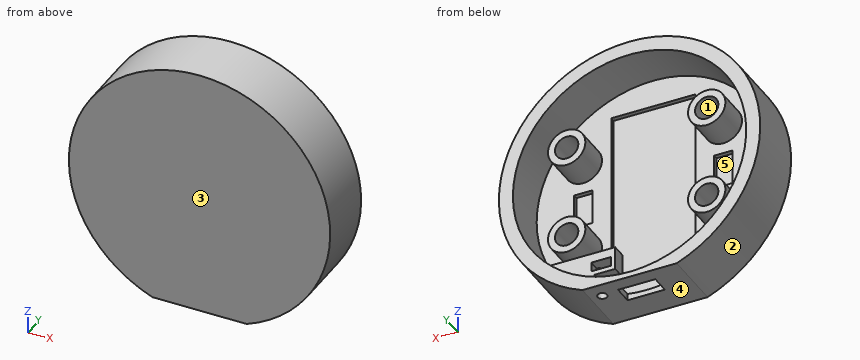
Autodesk Inventor part; units mm, degrees
ref_plane "YZ Plane" through (0, 0, 0) normal (1, 0, 0) x (0, 1, 0)
ref_plane "XZ Plane" through (0, 0, 0) normal (0, 1, 0) x (-1, 0, 0)
ref_plane "XY Plane" through (0, 0, 0) normal (0, 0, 1) x (1, 0, 0)
sketch "Sketch1" plane through (0, 0, 0) normal (0, 1, 0) x (-1, 0, 0)
  line L0 (8.5, 21.5) -> (-8.5, 21.5) construction
  line L1 (-8.5, 21.5) -> (-8.5, -21.5) construction
  line L2 (8.5, -21.5) -> (8.5, 21.5) construction
  line L3 (-8.5, 21.5) -> (8.5, -21.5) construction
  line L4 (-8.5, -21.5) -> (8.5, 21.5) construction
  line L5 (-3.5, -21.5) -> (-3.5, -23.5) construction
  line L6 (-3.5, -23.5) -> (3.5, -23.5) construction
  line L7 (3.5, -23.5) -> (3.5, -21.5) construction
  line L8 (-8.5, -21.5) -> (-3.5, -21.5) construction
  line L9 (3.5, -21.5) -> (8.5, -21.5) construction
  arc A0 (9.5253, -23.1034) -> (-9.5253, -23.1034) centre (0, 0) ccw
  line L10 (9.5253, -23.1034) -> (-9.5253, -23.1034)
  line L11 (-10.102, -26.1034) -> (10.102, -26.1034)
  arc A1 (10.102, -26.1034) -> (-10.102, -26.1034) centre (0, 0) ccw
  dimension "d0" = 43
  dimension "d1" = 17
  dimension "d2" = 7
  dimension "d3" = 2
  dimension "d4" = 3
  dimension "d13" = 20.204
extrude "BASE PLATE" add sketch "Sketch1" along normal blind 3 contours L10 A0 | A1 L11
sketch "Sketch3" plane through (0, 3, 0) normal (0, 1, 0) x (1, 0, 0)
  line L0 (10.102, 26.1034) -> (-10.102, 26.1034)
  arc A0 (-10.102, 26.1034) -> (10.102, 26.1034) centre (0, 0) ccw
  arc A1 (-10.102, 26.1034) -> (10.102, 26.1034) centre (0, 0) ccw
  line L1 (-10.102, 26.1034) -> (10.102, 26.1034)
  circle A2 centre (0, 0) radius 24.99
  dimension "d58" = 3
extrude "WALLS" add sketch "Sketch3" along normal blind 10
sketch "Sketch6" plane through (0, 3, 0) normal (0, 1, 0) x (1, 0, 0)
  line L0 (-8.5, 21.5) -> (8.5, 21.5) construction
  line L1 (8.5, 21.5) -> (8.5, -21.5) construction
  line L2 (8.5, -21.5) -> (-8.5, -21.5) construction
  line L3 (-8.5, -21.5) -> (-8.5, 21.5) construction
  line L4 (-8.5, -21.5) -> (8.5, 21.5) construction
  line L5 (-8.5, 21.5) -> (8.5, -21.5) construction
  line L6 (0, 0) -> (-15, 0) construction
  line L7 (-15, 0) -> (-15, 10) construction
  line L8 (-15, 10) -> (0, 10) construction
  line L9 (0, 10) -> (0, 0) construction
  circle A0 centre (-15, 10) radius 4
  circle A1 centre (-15, 10) radius 2.5
  circle A2 centre (-15, -10) radius 4
  circle A3 centre (-15, -10) radius 2.5
  circle A4 centre (15, 10) radius 4
  circle A5 centre (15, 10) radius 2.5
  circle A6 centre (15, -10) radius 2.5
  circle A7 centre (15, -10) radius 4
  dimension "d18" = 43
  dimension "d19" = 17
  dimension "d20" = 15
  dimension "d21" = 10
  dimension "d22" = 8
  dimension "d23" = 5
extrude "BUTTON POSTS" add sketch "Sketch6" along normal blind 7
sketch "Sketch7" plane through (0, 3, 0) normal (0, 1, 0) x (1, 0, 0)
  line L0 (-9, 24.1034) -> (9, 24.1034)
  line L1 (9, 24.1034) -> (9, -19.0966)
  line L2 (9, -19.0966) -> (-9, -19.0966)
  line L3 (-9, -19.0966) -> (-9, 24.1034)
  line L4 (-17, 3.75) -> (-13, 3.75)
  line L5 (-13, 3.75) -> (-13, -3.75)
  line L6 (-13, -3.75) -> (-17, -3.75)
  line L7 (-17, -3.75) -> (-17, 3.75)
  line L8 (-24.99, 0) -> (24.99, 0) construction
  line L9 (0, 23.1034) -> (0, -24.99) construction
  line L10 (17, 3.75) -> (13, 3.75)
  line L11 (13, 3.75) -> (13, -3.75)
  line L12 (13, -3.75) -> (17, -3.75)
  line L13 (17, -3.75) -> (17, 3.75)
  line L14 (-9.5253, 24.1034) -> (9.5253, 24.1034)
  line L15 (10.102, 26.1034) -> (-10.102, 26.1034)
  dimension "d26" = 43.2
  dimension "d27" = 18
  dimension "d28" = 7.5
  dimension "d29" = 4
  dimension "d30" = 3.75
  dimension "d63" = 2
  dimension "d65" = 9
  dimension "d77" = 13
extrude "INDENTATION FOR LINEUP" cut sketch "Sketch7" against normal blind 1
sketch "Sketch9" plane through (0, 2, 0) normal (0, 1, 0) x (1, 0, 0)
  line L0 (-9, 24.1034) -> (9, 24.1034)
  line L1 (-9, -19.0966) -> (9, -19.0966)
  line L2 (9, -19.0966) -> (9, 24.1034)
  line L3 (9, 24.1034) -> (-9, 24.1034)
  line L4 (-9, 24.1034) -> (-9, -19.0966)
  point P0 (0, 0)
extrude "FLAT SURFACE FOR ARDUINO" cut sketch "Sketch9" along normal blind 8
sketch "Sketch11" plane through (10.102, 0, -26.1034) normal (0, 0, -1) x (-1, 0, 0)
  line L0 (19.102, 2) -> (1.102, 2) construction
  line L1 (0, 0) -> (0, 13) construction
  line L2 (20.204, 0) -> (20.204, 13) construction
  line L3 (6.1, 10) -> (14.1, 10)
  line L4 (14.1, 10) -> (14.1, 6)
  line L5 (14.1, 6) -> (6.1, 6)
  line L6 (6.1, 6) -> (6.1, 10)
  line L7 (0, 0) -> (20.204, 0) construction
  circle A0 centre (2.5, 9.5) radius 1
  point P0 (10.102, 0)
  dimension "d69" = 4
  dimension "d70" = 4
  dimension "d71" = 6.1
  dimension "d72" = 2
  dimension "d74" = 2.5
  dimension "d78" = 7.5
  dimension "d89" = 8
extrude "I/O HOLES" cut sketch "Sketch11" against normal blind 10
sketch "Sketch12" plane through (0, 3, 0) normal (0, 1, 0) x (1, 0, 0)
  line L0 (19.1097, 16.1034) -> (9, 16.1034)
  line L1 (9, 16.1034) -> (9, 23.3131)
  line L2 (-9, 24.1034) -> (9, 24.1034) construction
  line L3 (-9, -19.0966) -> (-9, 24.1034) construction
  line L4 (9, -19.0966) -> (-9, -19.0966) construction
  line L5 (9, 24.1034) -> (9, -19.0966) construction
  line L6 (10.102, 26.1034) -> (-10.102, 26.1034)
  circle A0 centre (0, 0) radius 24.99 construction
  arc A1 (-9, 23.3131) -> (9, 23.3131) centre (0, 0) ccw
  arc A2 (19.1097, 16.1034) -> (9, 23.3131) centre (0, 0) ccw
  line L7 (9, 23.3131) -> (9, -19.0966)
  point P0 (13, 21.3424)
  dimension "d88" = 10
extrude "Extrusion11" add sketch "Sketch12" along normal blind 7
sketch "Sketch16" plane through (9, 2, -24.1034) normal (-1, 0, 0) x (0, 0, 1)
  line L0 (0, 8) -> (0, 6.5) construction
  line L1 (0.7903, 8) -> (8, 8) construction
  line L2 (6, 8) -> (6, 5.7) construction
  line L3 (6, 5.7) -> (4.3, 5.7) construction
  line L4 (4.3, 5.7) -> (4.3, 8) construction
  line L5 (0.7903, 8) -> (8, 8) construction
  line L6 (8, 1) -> (8, 8) construction
  line L7 (0.7903, 8) -> (8, 8) construction
  line L8 (14.8538, 7.25) -> (0, 7.25) construction
  line L9 (0, 0) -> (0, 8) construction
  line L10 (3, 8) -> (8, 8)
  line L11 (8, 8) -> (8, 5)
  line L12 (8, 5) -> (3, 5)
  line L13 (3, 5) -> (3, 8)
  point P0 (24.1034, -2)
  dimension "d96" = 3
  dimension "d97" = 5
extrude "Extrusion13" add sketch "Sketch16" along normal blind 4.398
sketch "Sketch18" plane through (0, 10, 0) normal (0, 1, 0) x (1, 0, 0)
  line L0 (9.727, 18.1034) -> (5.477, 18.1034)
  line L1 (5.477, 18.1034) -> (5.477, 20.1034)
  line L2 (5.477, 20.1034) -> (9.727, 20.1034)
  line L3 (9.727, 20.1034) -> (9.727, 18.1034)
  line L4 (19.1097, 16.1034) -> (4.602, 16.1034)
  line L5 (4.602, 16.1034) -> (4.602, 21.1034)
  line L6 (8.468, 23.5115) -> (8.468, 24.1034)
  line L7 (6.736, 24.1034) -> (6.736, 24.065)
  line L8 (8.468, 24.1034) -> (6.736, 24.1034)
  line L9 (6.602, 26.1034) -> (8.602, 26.1034)
  line L10 (7.602, 26.1034) -> (7.602, 13.109) construction
  point P0 (0, 0)
  dimension "d104" = 2
  dimension "d105" = 4.25
  dimension "d106" = 2
  dimension "d108" = 2.125
extrude "Extrusion15" cut sketch "Sketch18" against normal blind 2.3
sketch "Sketch20" plane through (0, 7.7, 0) normal (0, 1, 0) x (1, 0, 0)
  line L0 (9, 24.1034) -> (9, -19.0966)
  line L1 (5.477, 20.1034) -> (9.727, 20.1034)
  line L2 (5.477, 18.1034) -> (5.477, 20.1034)
  line L3 (9, 16.1034) -> (9, 21.1034)
  line L4 (9, 20.1034) -> (5.477, 20.1034)
  line L5 (5.477, 20.1034) -> (5.477, 18.1034)
  line L6 (5.477, 18.1034) -> (9, 18.1034)
  line L7 (9, 18.1034) -> (9, 20.1034)
  point P0 (0, 0)
extrude "Extrusion16" cut sketch "Sketch20" against normal up to next
equation "\"d30\" = 0.5 * d28"
equation "\"d65\" = 0.5 * d27"
equation "\"d108\" = 0.5 * d105"
properties part number "Base"
Verification items for the finished model (mm, model axes). Face numbers are marked on the shaded views. A direction names the side the tool comes from. Give positions to 0.01 mm unless a question says otherwise; leave off trailing zeros. Loops run counter-clockwise (first coordinate to the right, second up) from the corner with the lowest first, then second, coordinate; pieces in that order, holes last. Notation, with made-up numbers: M 89.25,28 L 100.25,28 A18 ccw 100.25,54 Z; hole C 76,64.5 d11. An arc over 180 degrees is marked long. Return JSON: item names as keys, results as strings.
1) Section check C-C, the plane z = 1.5. Enter the section's corners in (x, y), and give its area (3 significant figures).
Findings:
{"outline": "M -27.95,0 L 27.95,0 L 27.95,13 L 24.94,13 L 24.94,3 L 17,3 L 17,2 L 13,2 L 13,3 L 9,3 L 9,2 L -9,2 L -9,3 L -13,3 L -13,2 L -17,2 L -17,3 L -24.94,3 L -24.94,13 L -27.95,13 Z", "area": "202 mm2"}
2) Section check A-A, the plane y = 5.25. Count the separate pieces of the cut face and the enclosed holes in it, and give its area (3 significant figures).
Findings:
{"separate pieces": "5", "enclosed holes": "5", "area": "637 mm2"}
3) Section check D-D, the plane x = -15.5. Enter the section's corners in (y, z).
Findings:
{"outline": "M 0,-23.31 L 13,-23.31 L 13,-19.6 L 3,-19.6 L 3,-13.97 L 10,-13.97 L 10,-12.45 L 3,-12.45 L 3,-7.55 L 10,-7.55 L 10,-6.03 L 3,-6.03 L 3,-3.75 L 2,-3.75 L 2,3.75 L 3,3.75 L 3,6.03 L 10,6.03 L 10,7.55 L 3,7.55 L 3,12.45 L 10,12.45 L 10,13.97 L 3,13.97 L 3,19.6 L 13,19.6 L 13,23.31 L 0,23.31 Z"}
4) Tool access check on the marked faces 4 and 5. Record the directions out of +Z, -Z, +X, -X, +Y, -Y that give a thin tool (end or side, any length) a straight path to the whole face; none if there is none.
Findings:
{"face 4": "-Z, +X, -X, +Y, -Y", "face 5": "+Y"}
5) Gauge pin test, flat ends, axial feed: P1, Ø9, axis at x = 17, z = -8.5, coming from the +Y side; P2, Ø4, axis at x = 14, y = 5, coming from the -Z side; P3, Ø0.7, axis at y = 7, z = -25, coming from the +X side. Record the tip position at first contact, or that the pin passes through.
Findings:
{"P1": "stops at y = 10", "P2": "stops at z = -25.29", "P3": "stops at x = 13.26"}
6) Material ranges on L1, parallel to X at y = 9.5, z = -25.05; L2, parallel to Z at x = -0.5, y = 3.5 (1 decimal); L3, parallel to Z at x = 15, y = 5, recorded low to high. Write a range as [from, to].
Findings:
{"L1": "x = [-12.49, -4], [4, 6.6], [8.6, 12.49]", "L2": "z = [-26.1, -25], [25, 28]", "L3": "z = [-23.63, -16.1], [-14, -12.5], [-7.5, -6], [6, 7.5], [12.5, 14], [19.99, 23.63]"}
7) Mould release check, pull along X, two halves, no side actions. Record for the marked faces 1, 2 and 3: released by +X, released by -X, zero draft, split by the parting line, or undercut.
Findings:
{"face 1": "undercut", "face 2": "split by the parting line", "face 3": "zero draft"}
8) Section check B-B, the plane x = 0. Enter the section's corners in (y, z), and give its area (3 significant figures).
Findings:
{"outline": "M 0,-26.1 L 6,-26.1 L 6,-24.99 L 3,-24.99 L 3,-24.1 L 2,-24.1 L 2,19.1 L 3,19.1 L 3,24.99 L 13,24.99 L 13,27.99 L 0,27.99 Z; M 10,-26.1 L 13,-26.1 L 13,-24.99 L 10,-24.99 Z", "area": "156 mm2"}
